from build123d import *

# Parameters (mm, degrees)
BOSS_EXTRUDE1_DEPTH = 73.152
SKETCH2_R           = 14.351
CUT_EXTRUDE1_DEPTH  = 12.7
SKETCH3_R           = 18.415
CUT_EXTRUDE2_DEPTH  = 12.7
FILLET1_R           = 2.54


with BuildPart() as part:
    # Sketch1 → Boss-Extrude1 (new body)
    with BuildSketch(Plane.XY):
        Polygon((0, 0), (165.354, 0), (165.354, 73.152), (189.103, 73.152), (189.103, 0), (353.568, 0), (353.568, 3.175), (192.278, 3.175), (192.278, 76.327), (162.179, 76.327), (162.179, 3.175), (0, 3.175), align=None)
    extrude(amount=BOSS_EXTRUDE1_DEPTH)

    # Sketch2 → Cut-Extrude1 (cut)
    with BuildSketch(Plane.ZY.offset(-162.179)):
        with Locations((36.576, 25.146)):
            Circle(SKETCH2_R)
    extrude(amount=-CUT_EXTRUDE1_DEPTH, mode=Mode.SUBTRACT)

    # Sketch3 → Cut-Extrude2 (cut)
    with BuildSketch(Plane(origin=(192.278, 0, 0), x_dir=(0, 0, -1), z_dir=(1, 0, 0))):
        with Locations((-36.576, 25.146)):
            Circle(SKETCH3_R)
    extrude(amount=-CUT_EXTRUDE2_DEPTH, mode=Mode.SUBTRACT)

    # Fillet1
    fillet1_edges = [part.edges().sort_by_distance(p)[0] for p in [
        (162.179, 76.327, 36.576),
        (192.278, 76.327, 36.576),
        (189.103, 0, 36.576),
        (165.354, 0, 36.576),
    ]]
    fillet(fillet1_edges, radius=FILLET1_R)


solid = part.part
Design review of the part built by this model. Coordinates are the model's own, in mm. A direction names the side the tool comes from. Round coordinates to 2 decimals unless told otherwise and drop trailing zeros. Loops run counter-clockwise (first coordinate to the right, second up) from the corner with the lowest first, then second, coordinate; pieces in that order, holes last. Notation, with made-up numbers: (6, 66) - (51, 66) arc R13 ccw to (51, 84) - close; hole circle Ø6 at (61.5, 40). An arc over 180 degrees is marked (long way). One line per item, written item: value. Start each with the question number.
1) Consider section D-D on z = 68. Give the boundary of the cut face in (x, y) (3 decimals), then the cut area to 3 significant figures.
2) Insertion check: pin 1 Ø2 at (x, z) = (81.5, 30.5) entering from +Y (3 decimals); pin 2 Ø1.5 at (y, z) = (24.5, 56.5) entering from +X. Each pin has a flat end and moves straight along its axis. Give the tip position at first contact, or say it passes through.
3) Consider section C-C on y = 29. Give the boundary of the cut face in (x, z), then the cut area to 3 significant figures.
4) For faces 1 (the flat face through (192.278, 46, 36)), 2 (the flat face through (162.179, 47, 36)), 3 (the flat face through (189.103, 46, 36)), list the 3-axis set-ups (+Z, -Z, +X, -X, +Y, -Y) from which the entire face can be reached by the end or side of a thin tool; tool diameter is ignored.
5) To check wall thickness, follow L1, parallel to X at y = 58.5, z = 30.5; L2, parallel to X at y = 19.5, z = 52.5; L3, parallel to Y at x = 301.5, z = 27.5 (3 decimals). State the ranges of each line that lie inside material, in increasing order. Write a range as from..to.
6) Draft analysis for pull direction Y (two halves, no side actions). For faces 4 (the cylindrical face through (190.713, 18.093, 19.565)), 5 (the flat face through (163, 24, 0)), 6 (the flat face through (271, 0, 36)), state which applies: +Y half, -Y half, draft (parallel to the pull), parting line (faces both ways), or undercut.
7) Consider section B-B on z = 46.5. Give the boundary of the cut face in (x, y) (3 decimals).
8) Consider section A-A on y = 59.5. Give the boundary of the cut face in (x, z).
Reported:
1. outline: (0, 0) - (162.814, 0) arc R2.54 ccw to (165.354, 2.54) - (165.354, 73.152) - (189.103, 73.152) - (189.103, 2.54) arc R2.54 ccw to (191.643, 0) - (353.568, 0) - (353.568, 3.175) - (192.278, 3.175) - (192.278, 73.787) arc R2.54 ccw to (189.738, 76.327) - (164.719, 76.327) arc R2.54 ccw to (162.179, 73.787) - (162.179, 3.175) - (0, 3.175) - close
1. area: 1,580 mm^2
2. pin 1: stops at y = 3.175
2. pin 2: stops at x = 192.28
3. outline: (162.18, 0) - (165.35, 0) - (165.35, 22.75) - (162.18, 22.75) - close; (162.18, 50.4) - (165.35, 50.4) - (165.35, 73.15) - (162.18, 73.15) - close; (189.1, 0) - (192.28, 0) - (192.28, 18.57) - (189.1, 18.57) - close; (189.1, 54.58) - (192.28, 54.58) - (192.28, 73.15) - (189.1, 73.15) - close
3. area: 262 mm^2
4. face 1: +Z, -Z, +X, +Y
4. face 2: +Z, -Z, -X, +Y
4. face 3: +Z, -Z, -Y
5. L1: x = 162.18..165.35, 189.1..192.28
5. L2: x = 162.18..165.35
5. L3: y = 0..3.175
6. face 4: undercut
6. face 5: draft
6. face 6: -Y half
7. outline: (0, 0) - (162.814, 0) arc R2.54 ccw to (165.354, 2.54) - (165.354, 14.779) - (162.179, 14.779) - (162.179, 3.175) - (0, 3.175) - close; (162.179, 35.513) - (165.354, 35.513) - (165.354, 73.152) - (189.103, 73.152) - (189.103, 40.658) - (192.278, 40.658) - (192.278, 73.787) arc R2.54 ccw to (189.738, 76.327) - (164.719, 76.327) arc R2.54 ccw to (162.179, 73.787) - close; (189.103, 2.54) arc R2.54 ccw to (191.643, 0) - (353.568, 0) - (353.568, 3.175) - (192.278, 3.175) - (192.278, 9.634) - (189.103, 9.634) - close
8. outline: (162.18, 0) - (165.35, 0) - (165.35, 73.15) - (162.18, 73.15) - close; (189.1, 0) - (192.28, 0) - (192.28, 73.15) - (189.1, 73.15) - close
